```python
from build123d import *

# Parameters (mm, degrees)
SKETCH1_W           = 76.2
SKETCH1_H           = 69.85
SKETCH1_R           = 2.413
BOSS_EXTRUDE1_DEPTH = 3.175


with BuildPart() as part:
    # Sketch1 → Boss-Extrude1 (new body)
    with BuildSketch(Plane.XY):
        with Locations((38.1, 34.925)):
            Rectangle(SKETCH1_W, SKETCH1_H)
        with Locations((12.7, 59.69)):
            Circle(SKETCH1_R, mode=Mode.SUBTRACT)
        with Locations((38.1, 59.69)):
            Circle(SKETCH1_R, mode=Mode.SUBTRACT)
        with Locations((63.5, 59.69)):
            Circle(SKETCH1_R, mode=Mode.SUBTRACT)
        with Locations(Location((63.5, 10.16, 0), (0, 0, 180))):
            Circle(SKETCH1_R, mode=Mode.SUBTRACT)
        with Locations(Location((38.1, 10.16, 0), (0, 0, 180))):
            Circle(SKETCH1_R, mode=Mode.SUBTRACT)
        with Locations(Location((12.7, 10.16, 0), (0, 0, 180))):
            Circle(SKETCH1_R, mode=Mode.SUBTRACT)
    extrude(amount=BOSS_EXTRUDE1_DEPTH)


solid = part.part
```
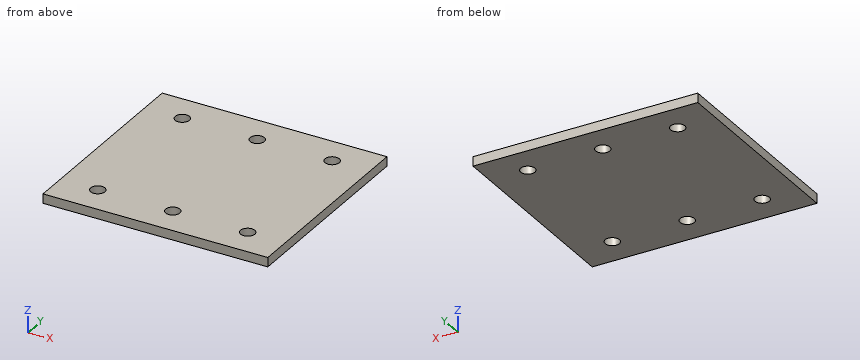
Here's how the part is built. I have some questions about the finished solid (model axes, mm). Coordinates: 2 decimals unless noted, no trailing zeros. Order: outer loops, then holes, each group sorted by start corner. A loop starts at its lowest first (then second) coordinate and runs counter-clockwise, first axis right, second up.
1) Imagine slicing it at A-A on y = 10.16. List the corners of the cut face in (x, z) for me (3 decimals).
2) Imagine slicing it at C-C on z = 0.9. List the corners of the cut face in (x, y) for me, and give its area (3 significant figures).
3) Will this pin go through, and if not, where does the flat tip stop? pin 1 (3 mm diameter, centred on x = 38.1, y = 10.16, fed in from -Z) (3 decimals).
4) I need wall thicknesses on line 1 (X direction, y = 10.16, z = 2.3); line 2 (Y direction, x = 63.5, z = 1.15); line 3 (Y direction, x = 12.5, z = 2.05). Which ranges of each line are inside material? Lowest first, please.
5) Imagine slicing it at B-B on x = 12.7. List the corners of the cut face in (y, z) for me (3 decimals).
Response values:
1. outline: (0, 0) - (10.287, 0) - (10.287, 3.175) - (0, 3.175) - close; (15.113, 0) - (35.687, 0) - (35.687, 3.175) - (15.113, 3.175) - close; (40.513, 0) - (61.087, 0) - (61.087, 3.175) - (40.513, 3.175) - close; (65.913, 0) - (76.2, 0) - (76.2, 3.175) - (65.913, 3.175) - close
2. outline: (0, 0) - (76.2, 0) - (76.2, 69.85) - (0, 69.85) - close; hole circle Ø4.83 at (12.7, 10.16); hole circle Ø4.83 at (12.7, 59.69); hole circle Ø4.83 at (38.1, 10.16); hole circle Ø4.83 at (38.1, 59.69); hole circle Ø4.83 at (63.5, 10.16); hole circle Ø4.83 at (63.5, 59.69)
2. area: 5,210 mm2
3. pin 1: passes through
4. line 1: x = 0 to 10.29, 15.11 to 35.69, 40.51 to 61.09, 65.91 to 76.2
4. line 2: y = 0 to 7.75, 12.57 to 57.28, 62.1 to 69.85
4. line 3: y = 0 to 7.76, 12.56 to 57.29, 62.09 to 69.85
5. outline: (0, 0) - (7.747, 0) - (7.747, 3.175) - (0, 3.175) - close; (12.573, 0) - (57.277, 0) - (57.277, 3.175) - (12.573, 3.175) - close; (62.103, 0) - (69.85, 0) - (69.85, 3.175) - (62.103, 3.175) - close
